```python
from build123d import *

# Parameters (mm, degrees)
F0_R     = 3.9882187516
F1_DEPTH = 3


with BuildPart() as f1:
    # F0 (on Front) → F1 (new body)
    with BuildSketch(Plane.XZ):
        with BuildLine():
            ThreePointArc((22.5, 16.15), (20.6401280605, 20.6401280605), (16.15, 22.5))
            Line((16.15, 22.5), (5.0711838848, 22.5))
            ThreePointArc((5.0711838848, 22.5), (0, 17.4288161152), (-5.0711838848, 22.5))
            Line((-5.0711838848, 22.5), (-16.15, 22.5))
            ThreePointArc((-16.15, 22.5), (-20.6401280605, 20.6401280605), (-22.5, 16.15))
            Line((-22.5, 16.15), (-22.5, -16.15))
            ThreePointArc((-22.5, -16.15), (-20.6401280605, -20.6401280605), (-16.15, -22.5))
            Line((-16.15, -22.5), (16.15, -22.5))
            ThreePointArc((16.15, -22.5), (20.6401280605, -20.6401280605), (22.5, -16.15))
            Line((22.5, -16.15), (22.5, 16.15))
        make_face()
        with Locations((0, -13.9503730461)):
            Circle(F0_R, mode=Mode.SUBTRACT)
        with BuildLine():
            Line((-5.0711838848, 22.5), (5.0711838848, 22.5))
            ThreePointArc((5.0711838848, 22.5), (0, 27.5711838848), (-5.0711838848, 22.5))
        make_face()
        with BuildLine():
            ThreePointArc((-5.0711838848, 22.5), (0, 17.4288161152), (5.0711838848, 22.5))
            Line((5.0711838848, 22.5), (-5.0711838848, 22.5))
        make_face()
    extrude(amount=F1_DEPTH)


solid = f1.part
```
The listing builds one solid part. Answer for the finished solid, in the listing's coordinates (mm). A direction names the side the tool comes from. Coordinates: 2 decimals unless noted, no trailing zeros. Write each loop counter-clockwise with the first axis right and the second up, starting at its lowest first coordinate (ties: lowest second). Pieces come first, ordered by that corner, then holes. Notation, with made-up numbers: (73, 22.5) -> (123, 22.5) arc R23 ccw to (123, 47.5) -> close; hole circle Ø6 at (32.25, -39). An arc over 180 degrees is marked (long way). Write each question's results on one line, items separated by ' | '. Start each with the question number.
1) Straight lines are drawn through the part: probe 1 along Z at (x, y) = (0, -1.7); probe 2 along Z at (x, y) = (12.5, -0.05); probe 3 along Z at (x, y) = (-2.5, -1.7). For each, find the intervals that lie inside material, in ascending order.
2) A cutting plane is placed at B-B (y = -0.7). Determine the outline of the cut face in (x, z), then the cut area to 3 significant figures.
3) A tool of negligible diameter and unlimited length cuts with its end or side. For faces 4 (the flat face through (-11, -1, 22.5)), 5 (the cylindrical face through (20.59, -1.48, -20.69)), from which of +Z, -Z, +X, -X, +Y, -Y can it reach the whole face along a straight path? Write none if from no direction.
4) A cutting plane is placed at C-C (x = -7). Determine the outline of the cut face in (y, z).
5) For a pull along X with two mould halves and no side action, classify faces 1 (the cylindrical face through (-0.865, -1.479, -17.844)), 2 (the cylindrical face through (-20.69, -1.48, -20.59)), 3 (the flat face through (11, -1, 22.5)) as +X half, -X half, draft (parallel to the pull), parting line (faces both ways), or undercut.
6) A cutting plane is placed at A-A (x = 0). Determine the outline of the cut face in (y, z).
7) A cutting plane is placed at D-D (z = 21). Determine the outline of the cut face in (x, y), then the cut area to 3 significant figures.
8) A flat-ended cylindrical pin translates along its axis: pin 1 Ø1.5 at (x, y) = (11, -2) entering from +Z. Find the tip coordinate at first contact, or state that the pin passes through.
Values follow:
1) probe 1: -22.5 to -17.94, -9.96 to 27.57 | probe 2: -22.5 to 22.5 | probe 3: -22.5 to -17.06, -10.84 to 26.91
2) outline: (-22.5, -16.15) arc R6.35 ccw to (-16.15, -22.5) -> (16.15, -22.5) arc R6.35 ccw to (22.5, -16.15) -> (22.5, 16.15) arc R6.35 ccw to (16.15, 22.5) -> (5.07, 22.5) arc R5.07 ccw to (-5.07, 22.5) -> (-16.15, 22.5) arc R6.35 ccw to (-22.5, 16.15) -> close; hole circle Ø7.98 at (0, -13.95) | area: 1,980 mm²
3) face 4: +Z, -X, +Y, -Y | face 5: -Z, +X, +Y, -Y
4) outline: (-3, -22.5) -> (0, -22.5) -> (0, 22.5) -> (-3, 22.5) -> close
5) face 1: undercut | face 2: -X half | face 3: draft
6) outline: (-3, -22.5) -> (0, -22.5) -> (0, -17.94) -> (-3, -17.94) -> close; (-3, -9.96) -> (0, -9.96) -> (0, 27.57) -> (-3, 27.57) -> close
7) outline: (-20.25, -3) -> (20.25, -3) -> (20.25, 0) -> (-20.25, 0) -> close | area: 121 mm²
8) pin 1: z = 22.5
